Autodesk Fusion 360 part; units mm, degrees
sketch "Sketch1" plane through (0, 0, 0) normal (0, 0, 1) x (1, 0, 0)
  line L0 (-41.91, -4.445) -> (41.91, -4.445)
  line L1 (41.91, -4.445) -> (41.91, 4.445)
  line L2 (41.91, 4.445) -> (-41.91, 4.445)
  line L3 (-41.91, 4.445) -> (-41.91, -4.445)
  line L4 (-41.91, 4.445) -> (41.91, -4.445) construction
  line L5 (41.91, 4.445) -> (-41.91, -4.445) construction
  dimension "d1" = 83.82
  dimension "d2" = 8.89
extrude "Extrude1" add sketch "Sketch1" along normal blind 4.7171 makes body 1
sketch "Sketch2" plane through (0, 0, 4.7171) normal (0, 0, 1) x (-1, 0, 0)
  line L0 (41.91, -4.445) -> (41.91, 4.445)
  line L1 (41.91, 4.445) -> (-41.91, 4.445)
  line L2 (-41.91, 4.445) -> (-41.91, -4.445)
  line L3 (-41.91, -4.445) -> (41.91, -4.445)
  line L4 (-41.91, -4.445) -> (41.91, -4.445)
  line L5 (41.91, -4.445) -> (41.91, -9.105)
  line L6 (41.91, -9.105) -> (-41.91, -9.105)
  line L7 (-41.91, -9.105) -> (-41.91, -4.445)
  line L8 (-41.91, -4.555) -> (41.91, -4.555)
  dimension "d5" = 4.66
  dimension "d34" = 0.11
extrude "Extrude2" add sketch "Sketch2" against normal blind 11.0067 separate body contours L5 L6 L7 L8 makes body 2
sketch "Sketch3" plane through (0, 0, 4.7171) normal (0, 0, 1) x (-1, 0, 0)
  line L0 (41.91, -4.445) -> (41.91, 4.445)
  line L1 (41.91, 4.445) -> (-41.91, 4.445)
  line L2 (-41.91, 4.445) -> (-41.91, -4.445)
  line L3 (-41.91, -9.105) -> (41.91, -9.105)
  line L4 (41.91, 4.445) -> (-41.91, 4.445)
  line L5 (-41.91, 4.445) -> (-41.91, 8.995)
  line L6 (-41.91, 8.995) -> (41.91, 8.995)
  line L7 (41.91, 8.995) -> (41.91, 4.445)
  line L8 (-41.91, -4.445) -> (41.91, -4.445)
  line L9 (-41.91, -4.555) -> (-41.91, -9.105)
  line L10 (41.91, -9.105) -> (41.91, -4.555)
  line L11 (41.91, -4.555) -> (-41.91, -4.555)
  dimension "d8" = 4.55
extrude "Extrude3" add sketch "Sketch3" against normal blind 16.51 contours L1 L4 L5 L6 L7 bodies 1
ref_plane "WorkPlane1" through (0, -2.275, -11.7929) normal (0, 0, 1) x (1, 0, 0)
sketch "Sketch4" plane through (0, 0, -11.7929) normal (0, 0, 1) x (1, 0, 0)
  line L0 (41.91, -8.995) -> (-41.91, -8.995)
  line L1 (-41.91, -8.995) -> (41.91, -8.995)
  line L2 (41.91, -8.995) -> (41.91, -38.995)
  line L3 (41.91, -38.995) -> (-41.91, -38.995)
  line L4 (-41.91, -38.995) -> (-41.91, -8.995)
  dimension "d12" = 30
extrude "Extrude4" add sketch "Sketch4" against normal blind 5 separate body makes body 3
sketch "Sketch5" plane through (0, 0, -11.7929) normal (0, 0, -1) x (1, 0, 0)
  line L0 (41.91, 8.995) -> (-41.91, 8.995)
  line L1 (-41.91, 8.995) -> (-41.91, 4.445)
  line L2 (-41.91, 4.445) -> (41.91, 4.445)
  line L3 (41.91, 4.445) -> (41.91, 8.995)
extrude "Extrude5" add sketch "Sketch5" along normal blind 5 bodies 1 3
extrude "Extrude6" add 1 faces at (13.97, -38.995, -13.4595) along direction (0, -1, 0) blind 8 on bodies 1 bodies 1
sketch "Sketch6" plane through (0, 0, -11.7929) normal (0, 0, 1) x (-1, 0, 0)
  line L0 (-41.91, 46.995) -> (-41.91, 8.995)
  line L1 (-41.91, 8.995) -> (41.91, 8.995)
  line L2 (41.91, 8.995) -> (41.91, 46.995)
  line L3 (6.3, 13.995) -> (-6.3, 13.995)
  line L4 (-6.3, 13.995) -> (-6.3, 41.995)
  line L5 (-6.3, 41.995) -> (6.3, 41.995)
  line L6 (6.3, 41.995) -> (6.3, 13.995)
  line L7 (6.3, 13.995) -> (-6.3, 41.995) construction
  line L8 (-6.3, 13.995) -> (6.3, 41.995) construction
  line L9 (-41.91, 8.995) -> (41.91, 8.995)
  line L10 (41.91, 46.995) -> (-41.91, 46.995)
  line L11 (11.3, 8.995) -> (-11.3, 8.995)
  line L12 (-11.3, 8.995) -> (-11.3, 46.995)
  line L13 (-11.3, 46.995) -> (11.3, 46.995)
  line L14 (11.3, 46.995) -> (11.3, 8.995)
  line L15 (0, 8.995) -> (0, 46.995) construction
  line L16 (16.3, 8.995) -> (-16.3, 8.995)
  line L17 (-16.3, 8.995) -> (-16.3, 46.995)
  line L18 (-16.3, 46.995) -> (16.3, 46.995)
  line L19 (16.3, 46.995) -> (16.3, 8.995)
  dimension "d17" = 12.6
  dimension "d18" = 28
  dimension "d22" = 5
  dimension "d23" = 5
  dimension "d24" = 5
  dimension "d25" = 5
  dimension "d26" = 5
  dimension "d27" = 25.61
extrude "Extrude7" cut 1 faces at (-41.91, -20.145, -15.1262) along direction (1, 0, 0) blind 25.61 on bodies 1 bodies 1
extrude "Extrude8" cut 1 faces at (41.91, -20.145, -15.1262) along direction (-1, 0, 0) blind 25.61 on bodies 1 bodies 1
extrude "Extrude9" add sketch "Sketch6" along normal blind 8.25 contours L1 L9 L10 L11 L12 L13 L14 L16 L18 bodies 1
extrude "Extrude10" add 1 faces at (5.4333, 4.445, 1.5724) along direction (0, 1, 0) blind 0.11 on bodies 1 bodies 1 2
extrude "Extrude11" cut 1 faces at (41.91, 7.5883, 1.0483) along direction (-1, 0, 0) blind 25.61 on bodies 1 bodies 1
extrude "Extrude12" cut 1 faces at (-41.91, 6.0717, 1.0483) along direction (1, 0, 0) blind 25.61 on bodies 1 bodies 1
equation "d3 = ( 33.02 / 7 ) * 1 mm"
equation "d6 = ( ( -2 * 33.02 ) / 6 ) * 1 mm"
equation "d9 = ( -33.02 / 2 ) * 1 mm"
equation "d11 = ( -33.02 / 2 ) * 1 mm"
equation "d32 = ( 33 / 4 ) * 1 mm"
Source: CAD feature listing. Evaluate the final solid. Frame: model axes, mm. A direction names the side the tool comes from. Coordinates: 2 decimals unless noted, no trailing zeros. Order: outer loops, then holes, each group sorted by start corner. A loop starts at its lowest first (then second) coordinate and runs counter-clockwise, first axis right, second up. Notation, with made-up numbers: M 64,-40 L 74,-40 A21 cw 74,-10 Z; hole C 68,79 d4. An arc over 180 degrees is marked long. Write each question's results on one line, items separated by ' | '. Start each with the question number.
1) Section query A-A (z = -4.5). Return the cut outline in (x, y) (3 decimals).
2) Draft query along X for faces 1 (the face through (-11.3, -28, -8)), 2 (the face through (0, -13.995, -8)), 3 (the face through (-14, -28, -11.793)). Return one class per face: released by +X, released by -X, zero draft, split by the parting line, or undercut.
3) Contact query for flat-ended pins moving along their axis: pin 1 Ø10 at (x, y) = (0, -32.5) entering from +Z; pin 2 Ø4 at (x, y) = (-13, -35.5) entering from +Z; pin 3 Ø1 at (x, z) = (-5.5, -7.5) entering from +Y (3 decimals); pin 4 Ø1.5 at (x, z) = (11, -3.5) entering from -Y (3 decimals). Output: stop coordinate, or through.
4) Section query D-D (z = -8.5). Return the cut outline in (x, y) (3 decimals).
5) Access query for faces 4 (the face through (0, 4.555, -3)), 5 (the face through (14, -28, -11.793)), 6 (the face through (-16.3, -15, -12)), 7 (the face through (0, 7, -6.29)), 8 (the face through (6.3, -28, -8)). Directions: +Z, -Z, +X, -X, +Y, -Y. A direction counts if a zero-diameter tool reaches every point of the face in a straight line with its end or side. Return the directions, or none.
6) Section query B-B (z = -1.25). Return the cut outline in (x, y) (3 decimals).
7) Section query C-C (x = -1.5). Return the cut outline in (y, z) (3 decimals).
8) Line query: line 1 (X direction, y = -18, z = -5.5); line 2 (Y direction, x = -7, z = -5.5) (3 decimals); line 3 (Y direction, x = 1.5, z = -8) (3 decimals). Output: solid intervals per line, ascending. Write a range as from..to.
Answers:
1) outline: M -16.3,-8.995 L -11.3,-8.995 L -11.3,-46.995 L 11.3,-46.995 L 11.3,-8.995 L 16.3,-8.995 L 16.3,-4.445 L -16.3,-4.445 Z; M -16.3,4.555 L 16.3,4.555 L 16.3,9.105 L -16.3,9.105 Z; hole M -6.3,-41.995 L 6.3,-41.995 L 6.3,-13.995 L -6.3,-13.995 Z
2) face 1: released by -X | face 2: undercut | face 3: zero draft
3) pin 1: stops at z = -11.79 | pin 2: stops at z = -3.54 | pin 3: stops at y = -4.445 | pin 4: stops at y = -46.995
4) outline: M -16.3,-8.995 L -11.3,-8.995 L -11.3,-46.995 L 11.3,-46.995 L 11.3,-8.995 L 16.3,-8.995 L 16.3,-4.445 L -16.3,-4.445 Z; hole M -6.3,-41.995 L 6.3,-41.995 L 6.3,-13.995 L -6.3,-13.995 Z
5) face 4: -Z, +X, -X | face 5: +Z, +X, -Y | face 6: +Z, -Z, -X, +Y, -Y | face 7: -Z, +X, -X, +Y | face 8: +Z
6) outline: M -16.3,-8.995 L 16.3,-8.995 L 16.3,-4.445 L -16.3,-4.445 Z; M -16.3,4.555 L 16.3,4.555 L 16.3,9.105 L -16.3,9.105 Z
7) outline: M -46.995,-16.793 L -4.445,-16.793 L -4.445,0 L 4.555,0 L 4.555,-6.29 L 9.105,-6.29 L 9.105,4.717 L -8.995,4.717 L -8.995,-3.543 L -13.995,-3.543 L -13.995,-11.793 L -41.995,-11.793 L -41.995,-3.543 L -46.995,-3.543 Z
8) line 1: x = -11.3..-6.3, 6.3..11.3 | line 2: y = -46.995..-4.445, 4.555..9.105 | line 3: y = -46.995..-41.995, -13.995..-4.445
